from build123d import *

# Parameters (mm, degrees)
SKETCH_1_W          = 16.3
SKETCH_1_H          = 44.96
EXTRUDE_1_DEPTH     = 2.27
SKETCH_2_W          = 13.16
SKETCH_2_H          = 39.68
CUT_EXTRUDE_1_DEPTH = 0.01
SKETCH_3_W          = 9
SKETCH_3_H          = 0.5
EXTRUDE_2_DEPTH     = 0.2
EXTRUDE_3_DEPTH     = 9
SKETCH_5_W          = 12.4
SKETCH_5_H          = 5.1
EXTRUDE_4_DEPTH     = 0.2
SKETCH_6_W          = 0.35
SKETCH_6_H          = 2
CUT_EXTRUDE_2_DEPTH = 0.05
FILLET_2_R          = 0.5


with BuildPart() as part:
    # 草图1 → 凸台-拉伸1 (new body)
    with BuildSketch(Plane(origin=(0, 0, 0), x_dir=(1, 0, 0), z_dir=(0, 1, 0))):
        Rectangle(SKETCH_1_W, SKETCH_1_H)
    extrude(amount=EXTRUDE_1_DEPTH)

    # 草图2 → 切除-拉伸1 (cut)
    with BuildSketch(Plane(origin=(0, 2.27, 0), x_dir=(1, 0, 0), z_dir=(0, 1, 0))):
        Rectangle(SKETCH_2_W, SKETCH_2_H)
    extrude(amount=-CUT_EXTRUDE_1_DEPTH, mode=Mode.SUBTRACT)

    # 草图3 → 凸台-拉伸2 (add)
    with BuildSketch(Plane(origin=(0, 1.27, 0), x_dir=(1, 0, 0), z_dir=(0, 1, 0))):
        with Locations((-0.25, -22.73)):
            Rectangle(SKETCH_3_W, SKETCH_3_H)
    extrude(amount=EXTRUDE_2_DEPTH)

    # 草图4 → 凸台-拉伸3 (add)
    with BuildSketch(Plane(origin=(4.25, 0, 0), x_dir=(0, 0, -1), z_dir=(1, 0, 0))):
        with BuildLine():
            Line((-22.73, 1.47), (-22.98, 1.47))
            ThreePointArc((-22.98, 1.47), (-24.615, -0.165), (-22.98, -1.8))
            Line((-22.98, -1.8), (-10.48, -1.8))
            Line((-10.48, -1.8), (-10.48, -1.6))
            Line((-10.48, -1.6), (-22.98, -1.6))
            ThreePointArc((-22.98, -1.6), (-24.415, -0.165), (-22.98, 1.27))
            Line((-22.98, 1.27), (-22.73, 1.27))
            Line((-22.73, 1.27), (-22.73, 1.47))
        make_face()
    extrude(amount=-EXTRUDE_3_DEPTH)

    # 草图5 → 凸台-拉伸4 (add)
    with BuildSketch(Plane.XZ.offset(1.8)):
        with Locations((-0.25, 13.03)):
            Rectangle(SKETCH_5_W, SKETCH_5_H)
    extrude(amount=-EXTRUDE_4_DEPTH)

    # 草图6 → 切除-拉伸2 (cut)
    with BuildSketch(Plane.XZ.offset(1.8)):
        with Locations((-4.45, 11.48)):
            Rectangle(SKETCH_6_W, SKETCH_6_H)
        with Locations((-3.75, 11.48)):
            Rectangle(SKETCH_6_W, SKETCH_6_H)
        with Locations((-3.05, 11.48)):
            Rectangle(SKETCH_6_W, SKETCH_6_H)
        with Locations((-2.35, 11.48)):
            Rectangle(SKETCH_6_W, SKETCH_6_H)
        with Locations((-1.65, 11.48)):
            Rectangle(SKETCH_6_W, SKETCH_6_H)
        with Locations((-0.95, 11.48)):
            Rectangle(SKETCH_6_W, SKETCH_6_H)
        with Locations((-0.25, 11.48)):
            Rectangle(SKETCH_6_W, SKETCH_6_H)
        with Locations((0.45, 11.48)):
            Rectangle(SKETCH_6_W, SKETCH_6_H)
        with Locations((1.15, 11.48)):
            Rectangle(SKETCH_6_W, SKETCH_6_H)
        with Locations((1.85, 11.48)):
            Rectangle(SKETCH_6_W, SKETCH_6_H)
        with Locations((2.55, 11.48)):
            Rectangle(SKETCH_6_W, SKETCH_6_H)
        with Locations((3.25, 11.48)):
            Rectangle(SKETCH_6_W, SKETCH_6_H)
        with Locations((3.95, 11.48)):
            Rectangle(SKETCH_6_W, SKETCH_6_H)
    extrude(amount=-CUT_EXTRUDE_2_DEPTH, mode=Mode.SUBTRACT)

    # 圆角2
    fillet_2_edges = [part.edges().sort_by_distance(p)[0] for p in [
        (-6.45, -1.7, 15.58),
        (5.95, -1.7, 10.48),
        (-4.75, -1.7, 15.58),
        (4.25, -1.7, 15.58),
        (-6.45, -1.7, 10.48),
        (5.95, -1.7, 15.58),
    ]]
    fillet(fillet_2_edges, radius=FILLET_2_R)


solid = part.part
Build history of the part. All positions in model axes, mm. A direction names the side the tool comes from. Round coordinates to 2 decimals unless told otherwise and drop trailing zeros. Write each loop counter-clockwise with the first axis right and the second up, starting at its lowest first coordinate (ties: lowest second). Pieces come first, ordered by that corner, then holes. Notation, with made-up numbers: M 76,29.5 L 102,29.5 A33 cw 102,57.5 Z; hole C 18.25,84 d7. An arc over 180 degrees is marked long. Use CSV: the item, a comma, the result in double quotes.
1. Two-plate mould, pull along Z, no slides. Class faces 3 (the face through (0, 0, 0)), 4 (the face through (-0.187, -0.197, 24.415)), 5 (the face through (0, 1, -22.48)): +Z half, -Z half, draft (parallel to the pull), parting line (faces both ways), or undercut.
Reply:
face 3,"draft"
face 4,"undercut"
face 5,"-Z half"
2. Flat gauge pins, fed straight in: pin 1 (3 mm diameter, centred on x = -3, z = -14.5, fed in from +Y); pin 2 (3 mm diameter, centred on x = 5, z = -1.5, fed in from -Y). Where does each tip first touch, or does it go through?
Reply:
pin 1,"stops at y = 2.26"
pin 2,"stops at y = 0"
3. Saw through at A-A (y = 0.85). Give the cut face in (x, z), plus the area to 3 significant figures.
Reply:
outline,"M -8.15,-22.48 L 8.15,-22.48 L 8.15,22.48 L -8.15,22.48 Z; M -4.75,23.99 L 4.25,23.99 L 4.25,24.26 L -4.75,24.26 Z"
area,"735 mm²"
4. Wall check: probe 1 along Y at (x, z) = (0.75, 16.5); probe 2 along Y at (x, z) = (3.5, -4.5); probe 3 along Z at (x, y) = (4, -0.15). Give the ranges that are in metal, low to high. Write a range as from..to.
Reply:
probe 1,"y = -1.8..-1.6, 0..2.26"
probe 2,"y = 0..2.26"
probe 3,"z = 24.41..24.61"
5. Tool access for faces 1 (the face through (0, -1.8, 17)), 2 (the face through (0, -1.6, 17)): list every direction of +Z, -Z, +X, -X, +Y, -Y with a clear straight run to the whole face (end or side of a thin tool).
Reply:
face 1,"+Z, -Z, +X, -X, -Y"
face 2,"-Z, +X, -X"
